Check sheet for the modelled part. Datum: model origin and axes. Units: mm. Face numbers are marked on the shaded views. A direction names the side the tool comes from. Round coordinates to 2 decimals unless told otherwise and drop trailing zeros. Order: outer loops, then holes, each group sorted by start corner. A loop starts at its lowest first (then second) coordinate and runs counter-clockwise, first axis right, second up. Notation, with made-up numbers: (68.25, -19) -> (88.25, -19) arc R14 cw to (88.25, 7) -> close; hole circle Ø6 at (77, -32). An arc over 180 degrees is marked (long way). Answer in a Markdown table with one row per item.
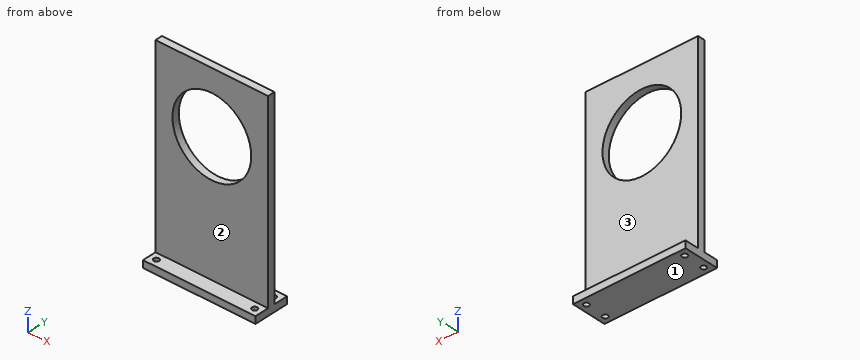
from build123d import *

# Parameters (mm, degrees)
F0_W     = 63.5
F0_H     = 107.95
F0_R     = 22.225
F1_DEPTH = 2
F2_W     = 63.5
F2_H     = 4
F3_DEPTH = 10
F4_R     = 1.5
F5_DEPTH = 25
F6_R     = 1.5
F7_DEPTH = 25


with BuildPart() as f1:
    # F0 (on Front) → F1 (new body, symmetric)
    with BuildSketch(Plane.XZ):
        with Locations((31.75, 53.975)):
            Rectangle(F0_W, F0_H)
        with Locations((31.75, 73.025)):
            Circle(F0_R, mode=Mode.SUBTRACT)
    extrude(amount=F1_DEPTH, both=True)

    # F2 (on Front) → F3 (join, symmetric)
    with BuildSketch(Plane.XZ):
        with Locations((31.75, -2)):
            Rectangle(F2_W, F2_H)
    extrude(amount=F3_DEPTH, both=True)

    # F4 (on face) → F5 (cut)
    with BuildSketch(Plane.XY):
        with Locations((4, 6)):
            Circle(F4_R)
        with Locations((59.5, 6)):
            Circle(F4_R)
    extrude(amount=-F5_DEPTH, mode=Mode.SUBTRACT)

    # F6 (on face) → F7 (cut)
    with BuildSketch(Plane.XY):
        with Locations((4, -6)):
            Circle(F6_R)
        with Locations((59.5, -6)):
            Circle(F6_R)
    extrude(amount=-F7_DEPTH, mode=Mode.SUBTRACT)


solid = f1.part
Item 1: Scan lines: line 1 (Y direction, x = 4, z = -3); line 2 (Y direction, x = 59, z = -2); line 3 (Y direction, x = 22, z = 102.5). Record each from-to range of solid material in increasing order. Write a range as [from, to].
Result sheet:
| item | result |
|---|---|
| line 1 | y = [-10, -7.5], [-4.5, 4.5], [7.5, 10] |
| line 2 | y = [-10, -7.41], [-4.59, 4.59], [7.41, 10] |
| line 3 | y = [-2, 2] |
Item 2: Cross-section at B-B (y = -6). Record the boundary of the cut face in (x, z), and give its area (3 significant figures).
Result sheet:
| item | result |
|---|---|
| outline | (0, -4) -> (2.5, -4) -> (2.5, 0) -> (0, 0) -> close; (5.5, -4) -> (58, -4) -> (58, 0) -> (5.5, 0) -> close; (61, -4) -> (63.5, -4) -> (63.5, 0) -> (61, 0) -> close |
| area | 230 mm^2 |
Item 3: Cross-section at C-C (x = 31.75). Record the boundary of the cut face in (y, z).
Result sheet:
| item | result |
|---|---|
| outline | (-10, -4) -> (10, -4) -> (10, 0) -> (2, 0) -> (2, 50.8) -> (-2, 50.8) -> (-2, 0) -> (-10, 0) -> close; (-2, 95.25) -> (2, 95.25) -> (2, 107.95) -> (-2, 107.95) -> close |
Item 4: Cross-section at A-A (x = 4). Record the boundary of the cut face in (y, z).
Result sheet:
| item | result |
|---|---|
| outline | (-10, -4) -> (-7.5, -4) -> (-7.5, 0) -> (-10, 0) -> close; (-4.5, -4) -> (4.5, -4) -> (4.5, 0) -> (2, 0) -> (2, 107.95) -> (-2, 107.95) -> (-2, 0) -> (-4.5, 0) -> close; (7.5, -4) -> (10, -4) -> (10, 0) -> (7.5, 0) -> close |
Item 5: Cross-section at D-D (z = 71). Record the boundary of the cut face in (x, y).
Result sheet:
| item | result |
|---|---|
| outline | (0, -2) -> (9.62, -2) -> (9.62, 2) -> (0, 2) -> close; (53.88, -2) -> (63.5, -2) -> (63.5, 2) -> (53.88, 2) -> close |
Item 6: Set-up check for the marked faces 1, 2 and 3: record each of +Z, -Z, +X, -X, +Y, -Y from which the full face is reachable in a straight line by a thin tool's end or side.
Result sheet:
| item | result |
|---|---|
| face 1 | -Z, +X, -X, +Y, -Y |
| face 2 | +Z, +X, -X, -Y |
| face 3 | +Z, +X, -X, +Y |
Item 7: Depth check by flat-ended pin: P1, Ø4, axis at x = 20, y = -7, coming from the +Z side; P2, Ø8, axis at x = 50, z = 68.5, coming from the -Y side; P3, Ø10, axis at x = 25.5, z = 48.5, coming from the +Y side. Enter the tip coordinate at first touch or a pass-through.
Result sheet:
| item | result |
|---|---|
| P1 | stops at z = 0 |
| P2 | stops at y = -2 |
| P3 | stops at y = 2 |
